Part model, mm, in its own coordinate system. A direction names the side the tool comes from. Round coordinates to 2 decimals unless told otherwise and drop trailing zeros. Order: outer loops, then holes, each group sorted by start corner. A loop starts at its lowest first (then second) coordinate and runs counter-clockwise, first axis right, second up. Notation, with made-up numbers: (-22.75, -1.75) -> (18.25, -1.75) arc R29 ccw to (18.25, 19.25) -> close; hole circle Ø5 at (-12.75, 87). An arc over 180 degrees is marked (long way). Use CSV: the item, a comma, the result in double quotes.
```python
from build123d import *

# Parameters (mm, degrees)
BOSS_EXTRUDE1_DEPTH = 6
BOSS_EXTRUDE2_DEPTH = 15
FILLET1_RADIUS      = 6
FILLET1_LENGTH      = 17
FILLET2_RADIUS      = 6
FILLET2_LENGTH      = 17
FILLET3_ANGLE       = 180
SKETCH2_R           = 3.5
CUT_EXTRUDE1_DEPTH  = 43.555845662


with BuildPart() as part:
    # Sketch1 → Boss-Extrude1 (new, symmetric)
    with BuildSketch(Plane(origin=(0, 0, 0), x_dir=(1, 0, 0), z_dir=(0, 1, 0))):
        with BuildLine():
            Line((25, 0), (23, 0))
            ThreePointArc((23, 0), (16.263455967, -16.263455967), (0, -23))
            Line((0, -23), (0, -31))
            Line((0, -31), (17, -31))
            Line((17, -31), (17, -18.33030278))
            ThreePointArc((17, -18.33030278), (22.912878475, -10), (25, 0))
        make_face()
        with BuildLine():
            Line((0, 31), (0, 23))
            ThreePointArc((0, 23), (16.263455967, 16.263455967), (23, 0))
            Line((23, 0), (25, 0))
            ThreePointArc((25, 0), (22.912878475, 10), (17, 18.33030278))
            Line((17, 18.33030278), (17, 31))
            Line((17, 31), (0, 31))
        make_face()
    extrude(amount=BOSS_EXTRUDE1_DEPTH, both=True)

    # Sketch1<4> → Boss-Extrude2 (add, symmetric)
    with BuildSketch(Plane(origin=(0, 0, 0), x_dir=(1, 0, 0), z_dir=(0, 1, 0))):
        with BuildLine():
            Line((0, 23), (0, 21))
            ThreePointArc((0, 21), (14.849242405, 14.849242405), (21, 0))
            Line((21, 0), (23, 0))
            ThreePointArc((23, 0), (16.263455967, 16.263455967), (0, 23))
        make_face()
        with BuildLine():
            Line((23, 0), (21, 0))
            ThreePointArc((21, 0), (14.849242405, -14.849242405), (0, -21))
            Line((0, -21), (0, -23))
            ThreePointArc((0, -23), (16.263455967, -16.263455967), (23, 0))
        make_face()
    extrude(amount=BOSS_EXTRUDE2_DEPTH, both=True)

    # Fillet1: full round fillet: the end face becomes a half cylinder, R = half its width
    fillet1_face = Plane((8.5, 0, 31), x_dir=(1, 0, 0), z_dir=(0, 0, 1))  # on the end face: x along it, z out of the body
    fillet1_slab = fillet1_face.offset(-FILLET1_RADIUS / 2) * Box(FILLET1_LENGTH, 2 * FILLET1_RADIUS, FILLET1_RADIUS, mode=Mode.PRIVATE)  # the body's end, R deep
    fillet1_round = Plane((8.5, 0, 25), x_dir=(0, 0, 1), z_dir=(1, 0, 0)) * Cylinder(FILLET1_RADIUS, FILLET1_LENGTH, mode=Mode.PRIVATE)  # its axis R under the face
    add(fillet1_slab - fillet1_round, mode=Mode.SUBTRACT)

    # Fillet2: full round fillet: the end face becomes a half cylinder, R = half its width
    fillet2_face = Plane((8.5, 0, -31), x_dir=(-1, 0, 0), z_dir=(0, 0, -1))  # on the end face: x along it, z out of the body
    fillet2_slab = fillet2_face.offset(-FILLET2_RADIUS / 2) * Box(FILLET2_LENGTH, 2 * FILLET2_RADIUS, FILLET2_RADIUS, mode=Mode.PRIVATE)  # the body's end, R deep
    fillet2_round = Plane((8.5, 0, -25), x_dir=(0, 0, -1), z_dir=(-1, 0, 0)) * Cylinder(FILLET2_RADIUS, FILLET2_LENGTH, mode=Mode.PRIVATE)  # its axis R under the face
    add(fillet2_slab - fillet2_round, mode=Mode.SUBTRACT)

    # Fillet3: read off the stored shape, not the designer's step
    # Fillet3 outline → Fillet3 (revolve)
    with BuildSketch(Plane.ZY):
        with BuildLine():
            ThreePointArc((23, -8), (23.585786438, -6.585786438), (25, -6))
            Line((25, -6), (23, -6))
            Line((23, -6), (23, -8))
        make_face()
        with BuildLine():
            Line((23, 6), (25, 6))
            ThreePointArc((25, 6), (23.585786438, 6.585786438), (23, 8))
            Line((23, 8), (23, 6))
        make_face()
    revolve(axis=Axis((0, 0, 0), (0, 1, 0)), revolution_arc=FILLET3_ANGLE)

    # Sketch2 → Cut-Extrude1 (cut, through all)
    with BuildSketch(Plane.ZY):
        with Locations((-26.5, 0)):
            Circle(SKETCH2_R)
        with Locations((26.5, 0)):
            Circle(SKETCH2_R)
    extrude(amount=-CUT_EXTRUDE1_DEPTH, mode=Mode.SUBTRACT)


solid = part.part
```
(1) Cut at C-C, the plane x = 10. State how many separate pieces and enclosed holes the cut face has, then the cut area to 3 significant figures.
Reply:
separate pieces,"2"
enclosed holes,"2"
area,"278 mm2"
(2) Pull direction Y, two halves, no side cores. Call faces 4 (the face through (0, 0.2, -22.6)), 5 (the face through (8.38, 1.05, 29.84)), 6 (the face through (9, 0, 31)): released by +Y, released by -Y, zero draft, split by the parting line, or undercut.
Reply:
face 4,"zero draft"
face 5,"undercut"
face 6,"split by the parting line"
(3) Which spindle directions (+Z, -Z, +X, -X, +Y, -Y) get a long thin tool onto all of the face, cutting with end or side? Do faces 1 (the face through (13, 6, -23)), 2 (the face through (17, 0, -22)), 3 (the face through (13, -6, -23)). Say none if no direction does.
Reply:
face 1,"-Z, +X, +Y"
face 2,"-Z, +X, +Y, -Y"
face 3,"-Z, +X, -Y"
(4) Drop flat-ended pins along their axis: P1, Ø3.5, axis at y = -0.5, z = 24, coming from the +X side; P2, Ø2, axis at x = 8.5, y = 10, coming from the +Z side; P3, Ø1.5, axis at x = 13.5, y = -10, coming from the +Z side. Give the stop position or say it passes through.
Reply:
P1,"x = 17"
P2,"z = 21.74"
P3,"z = 19.14"
(5) Probe probe 1 along Z at (x, y) = (13.25, -3); probe 2 along Y at (x, z) = (4.25, -26.5); probe 3 along Z at (x, y) = (1, 12). List the from-to ranges inside material, lowest first. Write a range as [from, to].
Reply:
probe 1,"[-30.2, -28.3], [-24.7, -16.29], [16.29, 24.7], [28.3, 30.2]"
probe 2,"[-5.81, -3.5], [3.5, 5.81]"
probe 3,"[-22.98, -20.98], [20.98, 22.98]"
(6) Cut at A-A, the plane y = 0. Give the cut face in (x, z), then the cut area to 3 significant figures.
Reply:
outline,"(0, -31) -> (17, -31) -> (17, -30) -> (0, -30) -> close; (0, -23) -> (17, -23) -> (17, -18.33) arc R25 ccw to (17, 18.33) -> (17, 23) -> (0, 23) -> (0, 21) arc R21 cw to (0, -21) -> close; (0, 30) -> (17, 30) -> (17, 31) -> (0, 31) -> close"
area,"326 mm2"
(7) Cut at B-B, the plane z = 26.5. Give the cut face in (x, y), then the cut area to 3 significant figures.
Reply:
outline,"(0, -5.81) -> (17, -5.81) -> (17, -3.5) -> (0, -3.5) -> close; (0, 3.5) -> (17, 3.5) -> (17, 5.81) -> (0, 5.81) -> close"
area,"78.5 mm2"
